from build123d import *

# Parameters (mm, degrees)
EXTRUDE_1_DEPTH     = 2
EXTRUDE_2_DEPTH     = 2
SKETCH_3_R          = 1
CUT_EXTRUDE_1_DEPTH = 2
CHAMFER_1_SIZE      = 2


with BuildPart() as part:
    # 草图1 → 凸台-拉伸1 (new body)
    with BuildSketch(Plane.XY):
        with BuildLine():
            Line((-20, -7), (-10.356157589, -7))
            ThreePointArc((-10.356157589, -7), (-12.5, 0), (-10.356157589, 7))
            Line((-10.356157589, 7), (-20, 7))
            Line((-20, 7), (-20, -7))
        make_face()
        with BuildLine():
            ThreePointArc((-10.356157589, -7), (-5.8630197, -11.039701083), (0, -12.5))
            Line((0, -12.5), (0, 12.5))
            ThreePointArc((0, 12.5), (-5.8630197, 11.039701083), (-10.356157589, 7))
            ThreePointArc((-10.356157589, 7), (-12.5, 0), (-10.356157589, -7))
        make_face()
        with BuildLine():
            Line((0, 12.5), (0, -12.5))
            ThreePointArc((0, -12.5), (5.8630197, -11.039701083), (10.356157589, -7))
            Line((10.356157589, -7), (10.356157589, 7))
            ThreePointArc((10.356157589, 7), (5.8630197, 11.039701083), (0, 12.5))
        make_face()
        with BuildLine():
            Line((10.356157589, 7), (10.356157589, -7))
            ThreePointArc((10.356157589, -7), (11.952028486, -3.66046651), (12.5, 0))
            ThreePointArc((12.5, 0), (11.952028486, 3.66046651), (10.356157589, 7))
        make_face()
        with BuildLine():
            ThreePointArc((12.5, 0), (11.952028486, -3.66046651), (10.356157589, -7))
            Line((10.356157589, -7), (20, -7))
            Line((20, -7), (20, 7))
            Line((20, 7), (10.356157589, 7))
            ThreePointArc((10.356157589, 7), (11.952028486, 3.66046651), (12.5, 0))
        make_face()
    extrude(amount=EXTRUDE_1_DEPTH)

    # 草图2 → 凸台-拉伸2 (add)
    with BuildSketch(Plane.ZY.offset(20)):
        with BuildLine():
            Line((28.9, 0), (2, 0))
            Line((2, 0), (2, -7))
            Line((2, -7), (30.34945143, -1.969234292))
            ThreePointArc((30.34945143, -1.969234292), (31.532792037, -1.284736771), (32, 0))
            Line((32, 0), (31.1, 0))
            ThreePointArc((31.1, 0), (30, -1.1), (28.9, 0))
        make_face()
        with BuildLine():
            Line((30.34945143, 1.969234292), (2, 7))
            Line((2, 7), (2, 0))
            Line((2, 0), (28.9, 0))
            ThreePointArc((28.9, 0), (30, 1.1), (31.1, 0))
            Line((31.1, 0), (32, 0))
            ThreePointArc((32, 0), (31.532792037, 1.284736771), (30.34945143, 1.969234292))
        make_face()
    extrude_2 = extrude(amount=-EXTRUDE_2_DEPTH)

    # 镜向1: 凸台-拉伸2 across plane
    add(extrude_2.mirror(Plane(origin=(0, 0, 0), x_dir=(0, 0, 1), z_dir=(1, 0, 0))))

    # 草图3 → 切除-拉伸1 (cut)
    with BuildSketch(Plane.XY.offset(2)):
        Circle(SKETCH_3_R)
        with BuildLine():
            Line((-11.5, 1), (-5.5, 1))
            ThreePointArc((-5.5, 1), (-4.5, 0), (-5.5, -1))
            Line((-5.5, -1), (-11.5, -1))
            ThreePointArc((-11.5, -1), (-12.5, 0), (-11.5, 1))
        make_face()
        with BuildLine():
            ThreePointArc((3.249191362, 8.927079897), (0, 9.5), (-3.249191362, 8.927079897))
            ThreePointArc((-3.249191362, 8.927079897), (-3.846863839, 7.645367133), (-2.565151075, 7.047694656))
            ThreePointArc((-2.565151075, 7.047694656), (0, 7.5), (2.565151075, 7.047694656))
            ThreePointArc((2.565151075, 7.047694656), (3.846863839, 7.645367133), (3.249191362, 8.927079897))
        make_face()
    cut_extrude_1 = extrude(amount=-CUT_EXTRUDE_1_DEPTH, mode=Mode.SUBTRACT)

    # 镜向2: 切除-拉伸1 across plane
    add(cut_extrude_1.mirror(Plane.ZX), mode=Mode.SUBTRACT)

    # 镜向3: 切除-拉伸1 across plane
    add(cut_extrude_1.mirror(Plane(origin=(0, 0, 0), x_dir=(0, 0, 1), z_dir=(1, 0, 0))), mode=Mode.SUBTRACT)

    # 倒角1
    chamfer_1_edges = [part.edges().sort_by_distance(p)[0] for p in [
        (-18, 0, 2),
        (18, 0, 2),
    ]]
    chamfer(chamfer_1_edges, length=CHAMFER_1_SIZE)


solid = part.part
Could you check a few things on this model? Use its own coordinates, in mm. A direction names the side the tool comes from. Give positions to 0.01 mm unless a question says otherwise; leave off trailing zeros. Order: outer loops, then holes, each group sorted by start corner. A loop starts at its lowest first (then second) coordinate and runs counter-clockwise, first axis right, second up.
Item 1: If we mould it in two halves opening along Y, with no side actions, what happens to faces 5 (the face through (9, 1, 1)), 6 (the face through (18.92, 4.45, 16.37)), 7 (the face through (-17, 0, 3))? For each: pulls with the +Y half, pulls with the -Y half, needs draft (parallel to the pull), parting line crosses it, or undercut.
Item 2: I need wall thicknesses on line 1 (X direction, y = 0, z = 0.65); line 2 (X direction, y = -2.25, z = 4.5); line 3 (Z direction, x = 14, y = 1). Which ranges of each line are inside material? Lowest first, please.
Item 3: For faces 1 (the face through (0, 9.5, 1)), 2 (the face through (15, 7, 1)), 3 (the face through (-18.92, 4.45, 16.37)), 4 (the face through (18, 0, 15)), which set-ups out of +Z, -Z, +X, -X, +Y, -Y let a thin tool reach every point of the face, with its end or its side?
Item 4: If we section it at D-D, the plane x = 14.5: Write out the boundary of the cut face in (y, z), plus the area to 3 significant figures.
Item 5: If we section it at C-C, the plane y = 3.25: Write out the boundary of the cut face in (x, z), plus the area to 3 significant figures.
Item 6: If we section it at B-B, the plane x = 7: Write out the boundary of the cut face in (y, z).
Item 7: I'm going to push flat-ended pins straight in: pin 1 (4 mm diameter, centred on x = 12.5, y = 2, fed in from -Z); pin 2 (1.6 mm diameter, centred on x = -9, z = 1, fed in from +Y); pin 3 (1 mm diameter, centred on x = 8, z = 1.5, fed in from +Y); pin 4 (2 mm diameter, centred on x = 15, z = 1.5, fed in from -Y). Where does each tip first touch, or does it pass through?
Item 8: If we section it at A-A, the plane z = 22: Write out the boundary of the cut face in (x, y), plus the area to 3 significant figures.
Values:
1. face 5: undercut
1. face 6: pulls with the +Y half
1. face 7: needs draft
2. line 1: x = -20 to -12.5, -4.5 to -1, 1 to 4.5, 12.5 to 20
2. line 2: x = -20 to -18, 18 to 20
2. line 3: z = 0 to 2
3. face 1: +Z, -Z
3. face 2: +Z, -Z, +X, +Y
3. face 3: +Z, +X, -X, +Y
3. face 4: +Z, +Y, -Y
4. outline: (-7, 0) - (7, 0) - (7, 2) - (-7, 2) - close
4. area: 28.0 mm2
5. outline: (-20, 0) - (20, 0) - (20, 23.13) - (18, 23.13) - (18, 4) - (16, 2) - (-16, 2) - (-18, 4) - (-18, 23.13) - (-20, 23.13) - close
5. area: 169 mm2
6. outline: (-10.36, 0) - (-1, 0) - (-1, 2) - (-10.36, 2) - close; (1, 0) - (10.36, 0) - (10.36, 2) - (1, 2) - close
7. pin 1: stops at z = 0
7. pin 2: stops at y = 9.43
7. pin 3: stops at y = 10
7. pin 4: stops at y = -7
8. outline: (-20, -3.45) - (-18, -3.45) - (-18, 3.45) - (-20, 3.45) - close; (18, -3.45) - (20, -3.45) - (20, 3.45) - (18, 3.45) - close
8. area: 27.6 mm2
